Source: CAD feature listing. Evaluate the final solid. Frame: model axes, mm. Coordinates: 2 decimals unless noted, no trailing zeros. Loops run counter-clockwise (first coordinate to the right, second up) from the corner with the lowest first, then second, coordinate; pieces in that order, holes last. Notation, with made-up numbers: (13.5, -31.75) -> (20.5, -31.75) arc R21 ccw to (20.5, 4.25) -> close; hole circle Ø3 at (84.25, -3.75). An arc over 180 degrees is marked (long way). One line per question, with ' | ' between items. Start each with the question number.
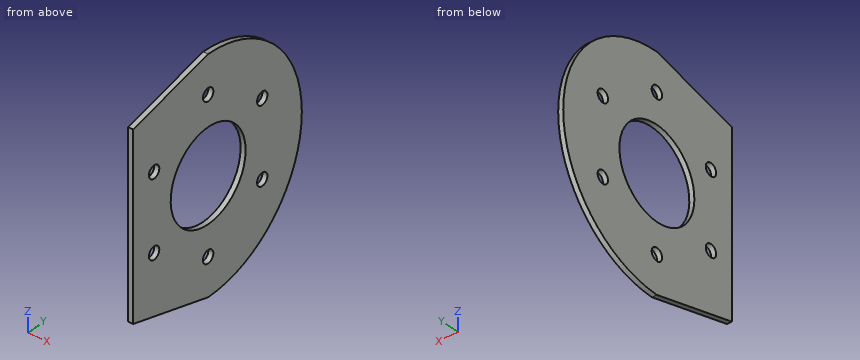
```python
from build123d import *

# Parameters (mm, degrees)
SKETCH1_R           = 9
BOSS_EXTRUDE1_DEPTH = 0.5
SKETCH2_R           = 1.25
CUT_EXTRUDE1_DEPTH  = 1


with BuildPart() as part:
    # Sketch1 → Boss-Extrude1 (new, symmetric)
    with BuildSketch(Plane(origin=(0, 0, 0), x_dir=(0, 0, -1), z_dir=(1, 0, 0))):
        with BuildLine():
            Line((-18, -18), (18, -18))
            Line((18, -18), (22.5, 0))
            ThreePointArc((22.5, 0), (0, 22.5), (-22.5, 0))
            Line((-22.5, 0), (-18, -18))
        make_face()
        Circle(SKETCH1_R, mode=Mode.SUBTRACT)
    extrude(amount=BOSS_EXTRUDE1_DEPTH, both=True)

    # Sketch2 → Cut-Extrude1 (cut)
    with BuildSketch(Plane(origin=(0.5, 0, 0), x_dir=(0, 0, -1), z_dir=(1, 0, 0))):
        with Locations((15, 0)):
            Circle(SKETCH2_R)
        with Locations((7.5, -12.990381057)):
            Circle(SKETCH2_R)
        with Locations((-7.5, -12.990381057)):
            Circle(SKETCH2_R)
        with Locations((-15, 0)):
            Circle(SKETCH2_R)
        with Locations((-7.5, 12.990381057)):
            Circle(SKETCH2_R)
        with Locations((7.5, 12.990381057)):
            Circle(SKETCH2_R)
    extrude(amount=-CUT_EXTRUDE1_DEPTH, mode=Mode.SUBTRACT)


solid = part.part
```
(1) Cut plane D-D, the plane x = -0.3. Return the cut outline in (y, z).
(2) Cut plane A-A, the plane z = 0. Return the cut outline in (x, y).
(3) Contact query for a flat-ended pin moving along its axis: pin 1 Ø2 at (y, z) = (0, -15) entering from +X. Output: stop coordinate, or through.
(4) Ray query, L1, parallel to Y at x = 0.2, z = -7.5; L2, parallel to Y at x = 0.05, z = 0; L3, parallel to Z at x = 0.2, y = 6.5. Return the intervals inside material, ascending.
(5) Cut plane B-B, the plane y = -6. Return the cut outline in (x, z).
(6) Cut plane C-C, the plane z = -7.5. Return the cut outline in (x, y), and give its area (3 significant figures).
Here are the results:
1) outline: (-18, -18) -> (0, -22.5) arc R22.5 ccw to (0, 22.5) -> (-18, 18) -> close; hole circle Ø2.5 at (-12.99, -7.5); hole circle Ø2.5 at (-12.99, 7.5); hole circle Ø18 at (0, 0); hole circle Ø2.5 at (0, -15); hole circle Ø2.5 at (0, 15); hole circle Ø2.5 at (12.99, -7.5); hole circle Ø2.5 at (12.99, 7.5)
2) outline: (-0.5, -18) -> (0.5, -18) -> (0.5, -9) -> (-0.5, -9) -> close; (-0.5, 9) -> (0.5, 9) -> (0.5, 22.5) -> (-0.5, 22.5) -> close
3) pin 1: passes through
4) L1: y = -18 to -14.24, -11.74 to -4.97, 4.97 to 11.74, 14.24 to 21.21 | L2: y = -18 to -9, 9 to 22.5 | L3: z = -21.54 to -6.22, 6.22 to 21.54
5) outline: (-0.5, -21) -> (0.5, -21) -> (0.5, -6.71) -> (-0.5, -6.71) -> close; (-0.5, 6.71) -> (0.5, 6.71) -> (0.5, 21) -> (-0.5, 21) -> close
6) outline: (-0.5, -18) -> (0.5, -18) -> (0.5, -14.24) -> (-0.5, -14.24) -> close; (-0.5, -11.74) -> (0.5, -11.74) -> (0.5, -4.97) -> (-0.5, -4.97) -> close; (-0.5, 4.97) -> (0.5, 4.97) -> (0.5, 11.74) -> (-0.5, 11.74) -> close; (-0.5, 14.24) -> (0.5, 14.24) -> (0.5, 21.21) -> (-0.5, 21.21) -> close | area: 24.3 mm2
